For this review, take the finished solid that the model builds, in its own axes (mm). Face numbers are marked on the shaded views. Give positions to 0.01 mm unless a question says otherwise; leave off trailing zeros. Order: outer loops, then holes, each group sorted by start corner. A loop starts at its lowest first (then second) coordinate and runs counter-clockwise, first axis right, second up. Notation, with made-up numbers: (-4.75, -19) -> (38.25, -19) arc R15 cw to (38.25, -5) -> close; hole circle Ø5 at (46, 57.5). An arc over 180 degrees is marked (long way). Return JSON: item names as keys, results as strings. Group by question number.
1) Add section D-D (x = 2.4). Give the boundary of the cut face in (y, z).
2) Add section C-C (y = -18). Give the boundary of the cut face in (x, z), then the cut area to 3 significant figures.
3) Insertion check: P1, Ø2.5, axis at y = -9, z = 15.59, coming from the +X side. The pin has a flat end and moves straight along its axis. Give the tip position at first contact, or say it passes through.
4) Add section B-B (z = 0). Give the boundary of the cut face in (x, y), then the cut area to 3 significant figures.
5) To check wall thickness, follow line 1 along Y through (x, z) = (1.25, 0); line 2 along Z through (x, y) = (2.55, 8); line 3 along Y through (x, z) = (0.55, -15.5). State the ranges of each line that lie inside material, in increasing order.
6) The part is to be moulded in two halves that separate along Z. For the marked faces 1, 2 and 3, say which applies: released by +Z, released by -Z, zero draft, split by the parting line, or undercut.
7) Add section A-A (y = 0). Give the boundary of the cut face in (x, z).
from build123d import *

# Parameters (mm, degrees)
SKETCH1_R          = 22.5
SKETCH1_R_2        = 11.2
EXTRUDE1_DEPTH     = 3
SKETCH2_R          = 1.5
CUT_EXTRUDE1_DEPTH = 4
CIRPATTERN1_COUNT  = 6


with BuildPart() as part:
    # Sketch1 → Extrude1 (new body)
    with BuildSketch(Plane(origin=(0, 0, 0), x_dir=(0, 0, -1), z_dir=(1, 0, 0))):
        Circle(SKETCH1_R)
        Circle(SKETCH1_R_2, mode=Mode.SUBTRACT)
    extrude(amount=EXTRUDE1_DEPTH)

    # Sketch2 → Cut-Extrude1 (cut, through all)
    with BuildSketch(Plane(origin=(3, 0, 0), x_dir=(0, 0, -1), z_dir=(1, 0, 0))):
        with Locations((0, 18)):
            Circle(SKETCH2_R)
    cut_extrude1 = extrude(amount=-CUT_EXTRUDE1_DEPTH, mode=Mode.SUBTRACT)

    # CirPattern1: Cut-Extrude1 ×6 about axis
    cirpattern1_axis = Axis((0, 0, 0), (1, 0, 0))
    for i in range(1, CIRPATTERN1_COUNT):
        add(cut_extrude1.rotate(cirpattern1_axis, i * 360 / CIRPATTERN1_COUNT), mode=Mode.SUBTRACT)


solid = part.part
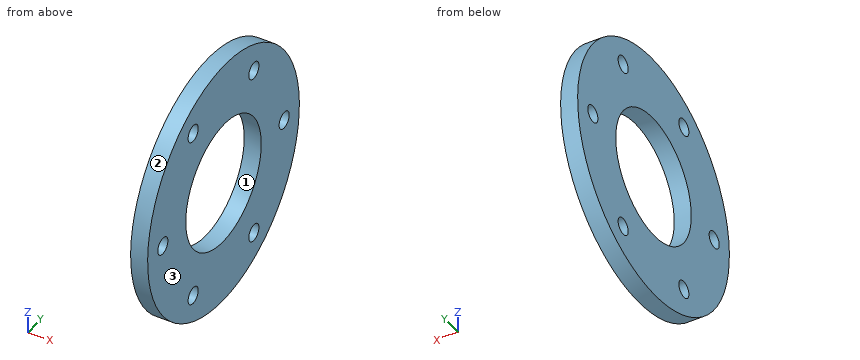
Evaluation:
{
 "1": {"outline": "circle Ø45 at (0, 0); hole circle Ø3 at (-18, 0); hole circle Ø22.4 at (0, 0); hole circle Ø3 at (-9, -15.59); hole circle Ø3 at (-9, 15.59); hole circle Ø3 at (9, -15.59); hole circle Ø3 at (9, 15.59); hole circle Ø3 at (18, 0)"},
 "2": {"outline": "(0, -13.5) -> (3, -13.5) -> (3, -1.5) -> (0, -1.5) -> close; (0, 1.5) -> (3, 1.5) -> (3, 13.5) -> (0, 13.5) -> close", "area": "72.0 mm^2"},
 "3": {"P1": "through"},
 "4": {"outline": "(0, -22.5) -> (3, -22.5) -> (3, -19.5) -> (0, -19.5) -> close; (0, -16.5) -> (3, -16.5) -> (3, -11.2) -> (0, -11.2) -> close; (0, 11.2) -> (3, 11.2) -> (3, 16.5) -> (0, 16.5) -> close; (0, 19.5) -> (3, 19.5) -> (3, 22.5) -> (0, 22.5) -> close", "area": "49.8 mm^2"},
 "5": {"line 1": "-22.5 to -19.5, -16.5 to -11.2, 11.2 to 16.5, 19.5 to 22.5", "line 2": "-21.03 to -16.71, -14.47 to -7.84, 7.84 to 14.47, 16.71 to 21.03", "line 3": "-16.31 to -10.5, -7.5 to 7.5, 10.5 to 16.31"},
 "6": {"face 1": "undercut", "face 2": "split by the parting line", "face 3": "zero draft"},
 "7": {"outline": "(0, -22.5) -> (3, -22.5) -> (3, -11.2) -> (0, -11.2) -> close; (0, 11.2) -> (3, 11.2) -> (3, 22.5) -> (0, 22.5) -> close"}
}
